Autodesk Inventor part; units mm, degrees
ref_plane "YZ Plane" through (0, 0, 0) normal (1, 0, 0) x (0, 1, 0)
ref_plane "XZ Plane" through (0, 0, 0) normal (0, 1, 0) x (-1, 0, 0)
ref_plane "XY Plane" through (0, 0, 0) normal (0, 0, 1) x (1, 0, 0)
sketch "Sketch1" plane through (0, 0, 0) normal (0, 0, 1) x (1, 0, 0)
  line L0 (-51.5762, 12.5065) -> (28.4238, 12.5065)
  line L1 (28.4238, 12.5065) -> (28.4238, -27.4935)
  line L2 (28.4238, -27.4935) -> (-51.5762, -27.4935)
  line L3 (-51.5762, -27.4935) -> (-51.5762, 12.5065)
  point P0 (0, 0)
  dimension "d0" = 80
  dimension "d1" = 40
extrude "Extrusion1" add sketch "Sketch1" along normal blind 2
sketch "Sketch2" plane through (0, 0, 2) normal (0, 0, 1) x (1, 0, 0)
  line L0 (-51.5762, 12.5065) -> (-51.5762, -27.4935)
  line L1 (-51.5762, -27.4935) -> (28.4238, -27.4935)
  point P0 (0, 0)
  point P1 (-44.5762, -14.4935)
  point P2 (2.2739, -14.4935)
  dimension "d4" = 46.8502
  dimension "d5" = 7
  dimension "d6" = 13
  dimension "d7" = 13
hole "Hole1" at (-44.5762, -14.4935, 2) at (2.2739, -14.4935, 2) direction (0, 0, -1) diameter 3 depth 8 tip angle 118
sketch "Sketch3" plane through (0, 0, 2) normal (0, 0, 1) x (1, 0, 0)
  point P0 (0, 0)
sketch "Sketch4" plane through (0, 0, 0) normal (0, 0, -1) x (-1, 0, 0)
  circle A0 centre (-2.2739, -14.4935) radius 1.5
  circle A1 centre (44.5762, -14.4935) radius 1.5
  circle A2 centre (-2.2739, 5.5065) radius 1.5
  circle A3 centre (44.5762, 5.5065) radius 1.5
  point P0 (0, 0)
  dimension "d15" = 20
  dimension "d16" = 20
  dimension "d17" = 3
  dimension "d18" = 3
extrude "Extrusion2" add sketch "Sketch4" along normal blind 7 contours A2 | A3
chamfer "Chamfer1" distance 2 angle 45 2 edges at (3.7739, 5.5065, 0) (-43.0762, 5.5065, 0)
properties part number "Power circuit support surface"
Could you check a few things on this model? Use its own coordinates, in mm. A direction names the side the tool comes from. Round coordinates to 2 decimals unless told otherwise and drop trailing zeros. Write each loop counter-clockwise with the first axis right and the second up, starting at its lowest first coordinate (ties: lowest second). Pieces come first, ordered by that corner, then holes. Notation, with made-up numbers: M 43,80 L 47,80 A29 cw 47,110 Z; hole C 23.5,7.5 d5. An arc over 180 degrees is marked long. Answer in a Markdown table with one row per item. Add a question column.
Q1. On a 3-axis mill with a long thin cutter (end or side, diameter ignored), from which of +Z, -Z, +X, -X, +Y, -Y can I reach the whole of each face in a straight line? I mean faces 4 (the cylindrical face through (2.6, 6.97, -4.46)), 5 (the cylindrical face through (3.187, -13.303, 0.986)). Say none if no direction works.
Q2. Imagine slicing it at A-A (y = -7.5). Please give me the cut outline in (x, z), then the cut area to 3 significant figures.
Q3. Imagine slicing it at C-C (x = 19). Please give me the cut outline in (y, z), then the cut area to 3 significant figures.
Q4. If I drill on line 1 (Z direction, x = -33.5, y = 7.5); line 2 (X direction, y = 6.5, z = -3); line 3 (X direction, y = 6.5, z = -0.75), over which ranges is the centre line in solid material (lowest first)? Write a range as from..to.
Q5. Imagine slicing it at B-B (z = -3). Please give me the cut outline in (x, y).
Q6. If we mould it in two halves opening along X, with no side actions, what happens to faces 1 (the flat face through (-51.576, -8, 1)), 2 (the cylindrical face through (-43.078, 5.441, -4.465)), 3 (the flat face through (-12, -7, 2))? For each: +X half, -X half, draft (parallel to the pull), parting line (faces both ways), or undercut.
Q7. Will these pins go through, and if not, where does the flat tip stop? pin 1 Ø12 at (x, y) = (-22.5, -11.5) entering from -Z; pin 2 Ø1.5 at (y, z) = (-10, -2.5) entering from +X; pin 3 Ø4 at (x, z) = (-42, -2.5) entering from -Y (3 decimals).
Values:
| question | item | result |
|---|---|---|
| 1 | face 4 | -Z |
| 1 | face 5 | +Z, -Z |
| 2 | outline | M -51.58,0 L 28.42,0 L 28.42,2 L -51.58,2 Z |
| 2 | area | 160 mm^2 |
| 3 | outline | M -27.49,0 L 12.51,0 L 12.51,2 L -27.49,2 Z |
| 3 | area | 80.0 mm^2 |
| 4 | line 1 | 0..2 |
| 4 | line 2 | -45.7..-43.45, 1.15..3.4 |
| 4 | line 3 | -47.14..-42.01, -0.29..4.84 |
| 5 | outline | C -44.58,5.51 d3; C 2.27,5.51 d3 |
| 6 | face 1 | -X half |
| 6 | face 2 | undercut |
| 6 | face 3 | draft |
| 7 | pin 1 | z = 0 |
| 7 | pin 2 | through |
| 7 | pin 3 | y = 3.275 |
